Build history of the part. All positions in model axes, mm. Face numbers are marked on the shaded views. A direction names the side the tool comes from. Coordinates: 2 decimals unless noted, no trailing zeros. Order: outer loops, then holes, each group sorted by start corner. A loop starts at its lowest first (then second) coordinate and runs counter-clockwise, first axis right, second up. Notation, with made-up numbers: (31.25, 52) -> (80.25, 52) arc R21 cw to (80.25, 80) -> close; hole circle Ø4 at (44, 27.25). An arc over 180 degrees is marked (long way). Write each question's results on one line, items separated by ' | '.
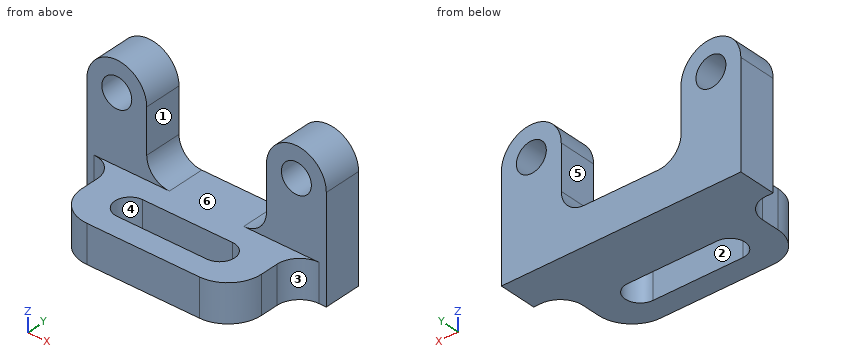
from build123d import *

# Parameters (mm, degrees)
F0_R     = 6.35
F1_DEPTH = 16.002
F2_R     = 9.652
F3_W     = 76.2
F3_H     = 31.496
F4_DEPTH = 16.002
F5_R     = 14.224
F6_R     = 9.652


with BuildPart() as f1:
    # F0 (on Front) → F1 (new body)
    with BuildSketch(Plane.XZ):
        with BuildLine():
            Line((-50.8, 44.45), (-50.8, 0))
            Line((-50.8, 0), (50.8, 0))
            Line((50.8, 0), (50.8, 44.45))
            ThreePointArc((50.8, 44.45), (38.1, 57.15), (25.4, 44.45))
            Line((25.4, 44.45), (25.4, 16.002))
            Line((25.4, 16.002), (-25.4, 16.002))
            Line((-25.4, 16.002), (-25.4, 44.45))
            ThreePointArc((-25.4, 44.45), (-38.1, 57.15), (-50.8, 44.45))
        make_face()
        with Locations((-38.1, 44.45)):
            Circle(F0_R, mode=Mode.SUBTRACT)
        with Locations((38.1, 44.45)):
            Circle(F0_R, mode=Mode.SUBTRACT)
    extrude(amount=-F1_DEPTH)

    # F2
    f2_edges = [f1.edges().sort_by_distance(p)[0] for p in [
        (-25.4, 8.001, 16.002),
        (25.4, 8.001, 16.002),
    ]]
    fillet(f2_edges, radius=F2_R)

    # F3 (on Top) → F4 (join)
    with BuildSketch(Plane.XY):
        with Locations((0, -15.748)):
            Rectangle(F3_W, F3_H)
        with BuildLine():
            ThreePointArc((-19.05, -22.098), (-25.4, -15.748), (-19.05, -9.398))
            Line((-19.05, -9.398), (19.05, -9.398))
            ThreePointArc((19.05, -9.398), (25.4, -15.748), (19.05, -22.098))
            Line((19.05, -22.098), (-19.05, -22.098))
        make_face(mode=Mode.SUBTRACT)
    extrude(amount=F4_DEPTH)

    # F5
    f5_edges = [f1.edges().sort_by_distance(p)[0] for p in [
        (38.1, -31.496, 8.001),
        (-38.1, -31.496, 8.001),
    ]]
    fillet(f5_edges, radius=F5_R)

    # F6
    f6_edges = [f1.edges().sort_by_distance(p)[0] for p in [
        (38.1, 0, 8.001),
        (-38.1, 0, 8.001),
    ]]
    fillet(f6_edges, radius=F6_R)


solid = f1.part
Item 1: Pin check, flat tips, straight feed: pin 1 (17.5 mm diameter, centred on x = -32.5, z = 23.5, fed in from -Y); pin 2 (10 mm diameter, centred on x = -38.1, z = 44.45, fed in from +Y); pin 3 (6 mm diameter, centred on y = -14, z = 4.5, fed in from -X); pin 4 (2.5 mm diameter, centred on y = -15, z = 10, fed in from +X). Stop position of each tip, or through.
Answer:
pin 1: stops at y = -30.89 | pin 2: passes through | pin 3: stops at x = -38.1 | pin 4: stops at x = 38.1
Item 2: Slice it at B-B, the plane y = 2. List the corners of the cut face in (x, z), and give its area (3 significant figures).
Answer:
outline: (-50.8, 0) -> (50.8, 0) -> (50.8, 44.45) arc R12.7 ccw to (25.4, 44.45) -> (25.4, 25.65) arc R9.65 cw to (15.75, 16) -> (-15.75, 16) arc R9.65 cw to (-25.4, 25.65) -> (-25.4, 44.45) arc R12.7 ccw to (-50.8, 44.45) -> close; hole circle Ø12.7 at (-38.1, 44.45); hole circle Ø12.7 at (38.1, 44.45) | area: 3,360 mm^2
Item 3: Slice it at C-C, the plane x = 3. List the corners of the cut face in (y, z), and give its area (3 significant figures).
Answer:
outline: (-31.5, 0) -> (-22.1, 0) -> (-22.1, 16) -> (-31.5, 16) -> close; (-9.4, 0) -> (16, 0) -> (16, 16) -> (-9.4, 16) -> close | area: 557 mm^2
Item 4: Slice it at D-D, the plane x = -34. List the corners of the cut face in (y, z).
Answer:
outline: (-27.26, 0) -> (16, 0) -> (16, 39.6) -> (0, 39.6) -> (0, 16) -> (-27.26, 16) -> close; (0, 49.3) -> (16, 49.3) -> (16, 56.47) -> (0, 56.47) -> close
Item 5: Tool access for the marked faces 4, 5 and 6: list every direction of +Z, -Z, +X, -X, +Y, -Y with a clear straight run to the whole face (end or side of a thin tool).
Answer:
face 4: +Z, -Z | face 5: +Z, +Y, -Y | face 6: +Z, -Y
Item 6: Pull direction Y, two halves, no side cores. Call the marked faces 1, 2 and 3: released by +Y, released by -Y, zero draft, split by the parting line, or undercut.
Answer:
face 1: zero draft | face 2: undercut | face 3: released by -Y
Item 7: Drill centre lines: line 1 (X direction, y = 6, z = 44); line 2 (Z direction, x = 38.1, y = 5.25); line 3 (X direction, y = 1, z = 41.5). Where is each one in solid material? Low to high. Write a range as from..to.
Answer:
line 1: x = -50.8..-44.43, -31.77..-25.4, 25.4..31.77, 44.43..50.8 | line 2: z = 0..38.1, 50.8..57.15 | line 3: x = -50.8..-43.72, -32.48..-25.4, 25.4..32.48, 43.72..50.8
Item 8: Slice it at A-A, the plane z = 32. List the corners of the cut face in (x, y).
Answer:
outline: (-50.8, 0) -> (-25.4, 0) -> (-25.4, 16) -> (-50.8, 16) -> close; (25.4, 0) -> (50.8, 0) -> (50.8, 16) -> (25.4, 16) -> close
